Read the model definition and answer for the solid it produces. Units are mm, in the model's axes. A direction names the side the tool comes from. Coordinates: 2 decimals unless noted, no trailing zeros. Order: outer loops, then holes, each group sorted by start corner. A loop starts at its lowest first (then second) coordinate and runs counter-clockwise, first axis right, second up.
```python
from build123d import *

# Parameters (mm, degrees)
BOSS_EXTRUDE1_DEPTH     = 10
CUT_EXTRUDE1_DEPTH      = 645.694266496
CUT_EXTRUDE1_DEPTH_BACK = 645.694266496
SKETCH3_R               = 3


with BuildPart() as part:
    # Sketch2 → Boss-Extrude1 (new body)
    with BuildSketch(Plane(origin=(707.562217201, 137.847000427, -295.175758868), x_dir=(0.354162422945148, 0.881836565444649, -0.31134105096888115), z_dir=(-0.9318848047050304, 0.30484147230294734, -0.1966275350098222))):
        Polygon((-166.545846492, -35.496085413), (-149.545846492, -35.496085413), (-149.545846492, -40.496085413), (-166.545846492, -40.496085413), (-166.545846492, -43.496085413), (-146.545846492, -43.496085413), (-146.545846492, -32.496085413), (-166.545846492, -32.496085413), align=None)
    extrude(amount=BOSS_EXTRUDE1_DEPTH)

    # Sketch3 → Cut-Extrude1 (cut, two sides: drawn at the far end of the back side and taken through both)
    with BuildSketch(Plane(origin=(18.826454002, -86.301151934, -223.021951761), x_dir=(-0.9969153981489656, -0.02832360582342947, -0.07319468755755801), z_dir=(0.07848368577920857, -0.35977207869560485, -0.9297334900161196)).offset(-CUT_EXTRUDE1_DEPTH_BACK)):
        with Locations(Location((-626.324876441, 87.720012572, 0), (0, 0, 90))):
            Circle(SKETCH3_R)
    extrude(amount=CUT_EXTRUDE1_DEPTH + CUT_EXTRUDE1_DEPTH_BACK, mode=Mode.SUBTRACT)


solid = part.part
```
1) A cutting plane is placed at A-A, the plane x = 638. Determine the outline of the cut face in (y, z).
A:
outline: (5.3, -214.8) - (8.94, -216.21) - (10.6, -213.63) - (6.3, -211.97) - close; (7.97, -207.23) - (13.38, -209.33) - (15.04, -206.74) - (8.97, -204.4) - close
2) A cutting plane is placed at D-D, the plane y = 12.25. State how many separate pieces and enclosed holes the cut face has, and give its area (3 significant figures).
A:
separate pieces: 4
enclosed holes: 0
area: 35.4 mm2
3) Flat-ended cylindrical pins translate along their axes: pin 1 Ø1 at (x, z) = (651, -213.5) entering from -Y; pin 2 Ø1 at (y, z) = (20.5, -205.5) entering from -X; pin 3 Ø1 at (y, z) = (10.5, -206.5) entering from -X; pin 4 Ø8 at (y, z) = (24.5, -212) entering from -X. Find the tip coordinate at first contact, or state that the pin passes through.
A:
pin 1: stops at y = 19.55
pin 2: passes through
pin 3: stops at x = 636.27
pin 4: stops at x = 640.65
4) A cutting plane is placed at C-C, the plane x = 649.75. Determine the outline of the cut face in (y, z), and give its area (3 significant figures).
A:
outline: (11.94, -216.38) - (21.41, -220.05) - (25.08, -209.64) - (18.05, -206.91) - (16.38, -209.5) - (21.09, -211.32) - (19.42, -216.05) - (13.61, -213.8) - close
area: 69.3 mm2
5) Determine the mould class of faces 1 (the flat face through (649.382, 11.999, -214.547)), 2 (the cylindrical face through (641.075, 12.132, -215.553)), 3 (the flat face through (646.06, 12.78, -217.02)) for opening direction Z: pulls with the +Z half, pulls with the -Z half, needs draft (parallel to the pull), parting line crosses it, or undercut.
A:
face 1: pulls with the +Z half
face 2: undercut
face 3: pulls with the -Z half
6) Straight lines are drawn through the part: line 1 (Z direction, x = 638.75, y = 9); line 2 (Y direction, x = 645, z = -212.5); line 3 (X direction, y = 24.75, z = -216.75). For each, find the intervals that lie inside material, in ascending order.
A:
line 1: z = -216.17 to -212.95, -207.57 to -204.34
line 2: y = 3.3 to 8.98, 22.58 to 25.98
line 3: x = 643.29 to 644.33
7) Which of the six approach directions +Z, -Z, +X, -X, +Y, -Y give full straight-line access (tool end or side, diameter ignored) to faces 4 (the flat face through (644.835, 14.311, -214.488)), 5 (the flat face through (641.317, 4.707, -212.705)), 6 (the flat face through (644.527, 16.319, -209.914))?
A:
face 4: -X
face 5: +Z, -X, -Y
face 6: none
8) A cutting plane is placed at B-B, the plane y = 18.25. Determine the outline of the cut face in (x, z).
A:
outline: (639.29, -207.88) - (639.96, -211.05) - (650.5, -210.16) - (649.83, -206.99) - close; (641.07, -216.33) - (641.74, -219.5) - (652.28, -218.61) - (651.62, -215.44) - close
